```python
from build123d import *

# Parameters (mm, degrees)
SKETCH_1_R               = 11.5
EXTRUDE_1_DEPTH          = 28
EXTRUDE_START            = -5
EXTRUDE_2_DEPTH          = 5
SKETCH_3_W               = 7
SKETCH_3_H               = 1
EXTRUDE_3_DEPTH          = 10
CHAMFER_1_SIZE           = 0.5
SKETCH_4_R               = 1
CUT_EXTRUDE_1_DEPTH      = 9
SKETCH_5_R               = 5.1
CUT_EXTRUDE_3_DEPTH      = 2
SKETCH_7_R               = 2
EXTRUDE_5_DEPTH          = 4
CUT_EXTRUDE_4_DEPTH      = 24
CUT_EXTRUDE_4_DEPTH_BACK = 4
CUT_EXTRUDE_5_DEPTH      = 24
CUT_EXTRUDE_5_DEPTH_BACK = 4


with BuildPart() as part:
    # Эскиз1 → Бобышка-Вытянуть1 (new body)
    with BuildSketch(Plane(origin=(0, 0, 0), x_dir=(1, 0, 0), z_dir=(0, 1, 0))):
        with Locations(Location((0, 0, 0), (0, 0, 270))):
            Circle(SKETCH_1_R)
    extrude(amount=EXTRUDE_1_DEPTH)

    # Эскиз2 → Бобышка-Вытянуть2 (add)
    with BuildSketch(Plane(origin=(0, 28, 0), x_dir=(1, 0, 0), z_dir=(0, 1, 0)).offset(EXTRUDE_START)):
        with BuildLine():
            Line((0, 11.5), (18.5, 11.5))
            Line((18.5, 11.5), (18.5, 2.5))
            Line((18.5, 2.5), (14.5, 2.5))
            Line((14.5, 2.5), (14.5, -2.5))
            Line((14.5, -2.5), (18.5, -2.5))
            Line((18.5, -2.5), (18.5, -11.5))
            Line((18.5, -11.5), (0, -11.5))
            ThreePointArc((0, -11.5), (11.5, 0), (0, 11.5))
        make_face()
    extrude(amount=EXTRUDE_2_DEPTH)

    # Эскиз3 → Бобышка-Вытянуть3 (add)
    with BuildSketch(Plane(origin=(18.5, 0, 0), x_dir=(0, 0, -1), z_dir=(1, 0, 0))):
        with Locations((-7, 25.5)):
            Rectangle(SKETCH_3_W, SKETCH_3_H)
        with Locations((7, 25.5)):
            Rectangle(SKETCH_3_W, SKETCH_3_H)
    extrude(amount=EXTRUDE_3_DEPTH)

    # Фаска1
    chamfer_1_edges = [part.edges().sort_by_distance(p)[0] for p in [
        (28.5, 25.5, 10.5),
        (28.5, 25.5, 3.5),
        (28.5, 25.5, -10.5),
        (28.5, 25.5, -3.5),
    ]]
    chamfer(chamfer_1_edges, length=CHAMFER_1_SIZE)

    # Эскиз4 → Вырез-Вытянуть1 (cut)
    with BuildSketch(Plane(origin=(0, 26, 0), x_dir=(1, 0, 0), z_dir=(0, 1, 0))):
        with Locations(Location((23.5, -7, 0), (0, 0, 270))):
            Circle(SKETCH_4_R)
        with Locations(Location((23.5, 7, 0), (0, 0, 270))):
            Circle(SKETCH_4_R)
    extrude(amount=-CUT_EXTRUDE_1_DEPTH, mode=Mode.SUBTRACT)

    # Эскиз5 → Вырез-Вытянуть3 (cut)
    with BuildSketch(Plane(origin=(0, 28, 0), x_dir=(1, 0, 0), z_dir=(0, 1, 0))):
        with Locations(Location((0, 0, 0), (0, 0, 270))):
            Circle(SKETCH_5_R)
    extrude(amount=-CUT_EXTRUDE_3_DEPTH, mode=Mode.SUBTRACT)

    # Эскиз7 → Бобышка-Вытянуть5 (add)
    with BuildSketch(Plane(origin=(0, 26, 0), x_dir=(1, 0, 0), z_dir=(0, 1, 0))):
        with Locations(Location((0, 0, 0), (0, 0, 270))):
            Circle(SKETCH_7_R)
        with BuildLine():
            Line((-3.570714214, 3.5), (-3.570714214, -3.5))
            ThreePointArc((-3.570714214, -3.5), (-5, 0), (-3.570714214, 3.5))
        make_face()
        with BuildLine():
            Line((3.5, 3.570714214), (-3.5, 3.570714214))
            ThreePointArc((-3.5, 3.570714214), (0, 5), (3.5, 3.570714214))
        make_face()
        with BuildLine():
            Line((3.570714214, -3.5), (3.570714214, 3.5))
            ThreePointArc((3.570714214, 3.5), (5, 0), (3.570714214, -3.5))
        make_face()
        with BuildLine():
            Line((-3.5, -3.570714214), (3.5, -3.570714214))
            ThreePointArc((3.5, -3.570714214), (0, -5), (-3.5, -3.570714214))
        make_face()
    extrude(amount=EXTRUDE_5_DEPTH)

    # Эскиз8 → Вырез-Вытянуть4 (cut, two sides: drawn at the far end of the back side and taken through both)
    with BuildSketch(Plane.ZY.offset(-3.570714214).offset(-CUT_EXTRUDE_4_DEPTH_BACK)):
        with BuildLine():
            Line((-3.5, 30), (-3.5, 29.75))
            ThreePointArc((-3.5, 29.75), (-3.426776695, 29.926776695), (-3.25, 30))
            Line((-3.25, 30), (-3.5, 30))
        make_face()
        with BuildLine():
            Line((3.25, 30), (3.5, 30))
            Line((3.5, 30), (3.5, 29.75))
            ThreePointArc((3.5, 29.75), (3.426776695, 29.926776695), (3.25, 30))
        make_face()
    extrude(amount=CUT_EXTRUDE_4_DEPTH + CUT_EXTRUDE_4_DEPTH_BACK, mode=Mode.SUBTRACT)

    # Эскиз9 → Вырез-Вытянуть5 (cut, two sides: drawn at the far end of the back side and taken through both)
    with BuildSketch(Plane.XY.offset(-3.570714214).offset(-CUT_EXTRUDE_5_DEPTH_BACK)):
        with BuildLine():
            Line((-3.5, 30), (-3.5, 29.75))
            ThreePointArc((-3.5, 29.75), (-3.426776695, 29.926776695), (-3.25, 30))
            Line((-3.25, 30), (-3.5, 30))
        make_face()
        with BuildLine():
            Line((3.25, 30), (3.5, 30))
            Line((3.5, 30), (3.5, 29.75))
            ThreePointArc((3.5, 29.75), (3.426776695, 29.926776695), (3.25, 30))
        make_face()
    extrude(amount=CUT_EXTRUDE_5_DEPTH + CUT_EXTRUDE_5_DEPTH_BACK, mode=Mode.SUBTRACT)


solid = part.part
```
Could you check a few things on this model? Use its own coordinates, in mm. A direction names the side the tool comes from. Round coordinates to 2 decimals unless told otherwise and drop trailing zeros. Loops run counter-clockwise (first coordinate to the right, second up) from the corner with the lowest first, then second, coordinate; pieces in that order, holes last. Notation, with made-up numbers: (59.5, -34) - (106.5, -34) arc R9 ccw to (106.5, -19) - close; hole circle Ø5 at (0.5, 69). An arc over 180 degrees is marked (long way). Answer in a Markdown table with one row per item. Add a question column.
(1) For faces 4 (the face through (22, 26, -7)), 5 (the face through (9, 25, -11.5)), 6 (the face through (16, 25, 2.5)), 7 (the face through (7, 28, 0)), 8 (the face through (-4, 30, 0)), which set-ups out of +Z, -Z, +X, -X, +Y, -Y let a thin tool reach every point of the face, with its end or its side?
(2) If we mould it in two halves opening along X, with no side actions, what happens to faces 1 (the face through (4, 30, 0)), 2 (the face through (14.5, 25, 0)), 3 (the face through (5, 28.4, -0.1))? For each: pulls with the +X half, pulls with the -X half, needs draft (parallel to the pull), parting line crosses it, or undercut.
(3) If we section it at B-B (x = 23.5): Please give me the cut outline in (y, z).
(4) If we section it at D-D (x = 1.5): Please give me the cut outline in (y, z), plus the area to 3 significant figures.
(5) If we section it at C-C (z = 0): Please give me the cut outline in (x, y).
(6) I'm going to push flat-ended pins straight in: pin 1 (7.5 mm diameter, centred on x = 22.5, z = 8.5, fed in from -Y); pin 2 (3 mm diameter, centred on x = 23.5, z = -7, fed in from +Y); pin 3 (8 mm diameter, centred on x = 24, y = 25.5, fed in from +Z). Where does each tip first touch, or does it pass through?
(7) I need wall thicknesses on line 1 along Y through (x, z) = (16, 7.25); line 2 along Y through (x, z) = (-9, -3.5); line 3 along X through (y, z) = (25.4, 7). Which ranges of each line are inside material? Lowest first, please.
(8) If we section it at A-A (z = 7): Please give me the cut outline in (x, y), plus the area to 3 significant figures.
Model answer:
| question | item | result |
|---|---|---|
| 1 | face 4 | +Z, -Z, +X, +Y |
| 1 | face 5 | -Z, +X, -X, +Y, -Y |
| 1 | face 6 | +X, +Y, -Y |
| 1 | face 7 | +Y |
| 1 | face 8 | +Z, -Z, +X, -X, +Y |
| 2 | face 1 | needs draft |
| 2 | face 2 | pulls with the +X half |
| 2 | face 3 | undercut |
| 3 | outline | (25, -10.5) - (26, -10.5) - (26, -8) - (25, -8) - close; (25, -6) - (26, -6) - (26, -3.5) - (25, -3.5) - close; (25, 3.5) - (26, 3.5) - (26, 6) - (25, 6) - close; (25, 8) - (26, 8) - (26, 10.5) - (25, 10.5) - close |
| 4 | outline | (0, -11.4) - (23, -11.4) - (23, -11.5) - (28, -11.5) - (28, -4.87) - (26, -4.87) - (26, -4.77) - (30, -4.77) - (30, -3.57) - (26, -3.57) - (26, -1.32) - (30, -1.32) - (30, 1.32) - (26, 1.32) - (26, 3.57) - (30, 3.57) - (30, 4.77) - (26, 4.77) - (26, 4.87) - (28, 4.87) - (28, 11.5) - (23, 11.5) - (23, 11.4) - (0, 11.4) - close |
| 4 | area | 640 mm² |
| 5 | outline | (-11.5, 0) - (11.5, 0) - (11.5, 23) - (14.5, 23) - (14.5, 28) - (5.1, 28) - (5.1, 26) - (5, 26) - (5, 30) - (3.57, 30) - (3.57, 26) - (2, 26) - (2, 30) - (-2, 30) - (-2, 26) - (-3.57, 26) - (-3.57, 30) - (-5, 30) - (-5, 26) - (-5.1, 26) - (-5.1, 28) - (-11.5, 28) - close |
| 6 | pin 1 | stops at y = 25 |
| 6 | pin 2 | stops at y = 26 |
| 6 | pin 3 | stops at z = 10.5 |
| 7 | line 1 | y = 23 to 28 |
| 7 | line 2 | y = 0 to 28 |
| 7 | line 3 | x = -9.12 to 22.5, 24.5 to 28.5 |
| 8 | outline | (-9.12, 0) - (9.12, 0) - (9.12, 23) - (18.5, 23) - (18.5, 25) - (22.5, 25) - (22.5, 26) - (18.5, 26) - (18.5, 28) - (-9.12, 28) - close; (24.5, 25) - (28.5, 25) - (28.5, 26) - (24.5, 26) - close |
| 8 | area | 566 mm² |
